The model under review builds one solid part; all positions refer to its coordinate system, in mm. A direction names the side the tool comes from. Coordinates: 2 decimals unless noted, no trailing zeros. Order: outer loops, then holes, each group sorted by start corner. A loop starts at its lowest first (then second) coordinate and runs counter-clockwise, first axis right, second up. Notation, with made-up numbers: (17, 75) -> (48, 75) arc R21 cw to (48, 96) -> close; hole circle Ø9 at (-0.5, -22.75). An arc over 180 degrees is marked (long way). Use one line per item in the form item = value.
from build123d import *

# Parameters (mm, degrees)
SKETCH1_R           = 12.7
BOSS_EXTRUDE1_DEPTH = 12.7
BOSS_EXTRUDE1_DRAFT = -5
SKETCH2_R           = 3.175
CUT_EXTRUDE1_DEPTH  = 22.997045256
SKETCH7_R           = 1.27
CUT_EXTRUDE2_DEPTH  = 7.62


with BuildPart() as part:
    # Sketch1 → Boss-Extrude1 (with draft: the straight prism first)
    with BuildSketch(Plane(origin=(0, 0, 0), x_dir=(1, 0, 0), z_dir=(0, 1, 0))):
        Circle(SKETCH1_R)
    extrude(amount=-BOSS_EXTRUDE1_DEPTH)
    # Boss-Extrude1: the draft: its side faces are tilted about the plane it starts from
    boss_extrude1_sides = [part.faces().sort_by_distance(p)[0] for p in [
        (-12.7, -6.35, 0),
    ]]
    draft(boss_extrude1_sides, Plane(origin=(0, 0, 0), x_dir=(1, 0, 0), z_dir=(0, 1, 0)), BOSS_EXTRUDE1_DRAFT)

    # Sketch2 → Cut-Extrude1 (cut, through all)
    with BuildSketch(Plane(origin=(0, 0, 0), x_dir=(1, 0, 0), z_dir=(0, 1, 0))):
        with Locations(Location((0, 0, 0), (0, 0, 270))):
            Circle(SKETCH2_R)
    extrude(amount=-CUT_EXTRUDE1_DEPTH, mode=Mode.SUBTRACT)

    # Sketch7 → Cut-Extrude2 (cut)
    with BuildSketch(Plane.XZ.offset(12.7)):
        with Locations(Location((-8.636, 0, 0), (0, 0, 270))):
            Circle(SKETCH7_R)
        with Locations(Location((4.318, 7.478995387, 0), (0, 0, 270))):
            Circle(SKETCH7_R)
    extrude(amount=-CUT_EXTRUDE2_DEPTH, mode=Mode.SUBTRACT)


solid = part.part
Item 1: Draft analysis for pull direction X (two halves, no side actions). For faces 1 (the face through (3, 0, 3)), 2 (the face through (-1.566, -7.672, -11.926)), 3 (the face through (3.55, -8.94, 8.49)), state which applies: released by +X, released by -X, zero draft, split by the parting line, or undercut.
Results found:
face_1 = zero draft
face_2 = split by the parting line
face_3 = undercut
Item 2: We need section C-C (y = -8.5). Write out the cut boundary in (x, z) (3 decimals).
Results found:
outline = circle Ø23.913 at (0, 0); hole circle Ø2.54 at (-8.636, 0); hole circle Ø6.35 at (0, 0); hole circle Ø2.54 at (4.318, 7.479)
Item 3: We need section B-B (x = 0). Write out the cut boundary in (y, z) (3 decimals), plus the area to 3 significant figures.
Results found:
outline = (-12.7, -11.589) -> (0, -12.7) -> (0, -3.175) -> (-12.7, -3.175) -> close; (-12.7, 3.175) -> (0, 3.175) -> (0, 12.7) -> (-12.7, 11.589) -> close
area = 228 mm²
Item 4: We need section A-A (z = 0). Write out the cut boundary in (x, y) (3 decimals).
Results found:
outline = (-12.7, 0) -> (-11.589, -12.7) -> (-9.906, -12.7) -> (-9.906, -5.08) -> (-7.366, -5.08) -> (-7.366, -12.7) -> (-3.175, -12.7) -> (-3.175, 0) -> close; (3.175, -12.7) -> (11.589, -12.7) -> (12.7, 0) -> (3.175, 0) -> close
Item 5: We need section D-D (y = -4.25). Write out the cut boundary in (x, z) (3 decimals).
Results found:
outline = circle Ø24.656 at (0, 0); hole circle Ø6.35 at (0, 0)
Item 6: Clearance check with flat-ended pins moving along their axes: pin 1 (3.5 mm diameter, centred on x = 4.32, z = 7.48, fed in from -Y); pin 2 (1.5 mm diameter, centred on x = -3, y = -4.5, fed in from +Z); pin 3 (5 mm diameter, centred on x = 0, z = 0, fed in from +Y); pin 4 (1 mm diameter, centred on y = -9, z = -3, fed in from -X). State where each tip first meets the part, or that it passes through.
Results found:
pin_1 = -12.7
pin_2 = 12.11
pin_3 = through
pin_4 = -11.66
Item 7: Tool access review of faces 4 (the face through (4, -5.08, 7)), 5 (the face through (-1.93, -6.26, -2.52)): name each direction out of +Z, -Z, +X, -X, +Y, -Y from which nothing blocks a thin tool from reaching the whole face with its end or side.
Results found:
face_4 = -Y
face_5 = +Y, -Y
Item 8: To check wall thickness, follow L1, parallel to X at y = -5.25, z = 0 (3 decimals); L2, parallel to X at y = -9.75, z = 8; L3, parallel to Z at x = 2.75, y = -1.25. State the ranges of each line that lie inside material, in increasing order. Write a range as from..to.
Results found:
L1 = -12.241..-9.906, -7.366..-3.175, 3.175..12.241
L2 = -8.74..3.16, 5.48..8.74
L3 = -12.29..-1.59, 1.59..12.29
